Read the model definition and answer for the solid it produces. Units are mm, in the model's axes. A direction names the side the tool comes from. Coordinates: 2 decimals unless noted, no trailing zeros. Order: outer loops, then holes, each group sorted by start corner. A loop starts at its lowest first (then second) coordinate and runs counter-clockwise, first axis right, second up. Notation, with made-up numbers: (11.25, 67) -> (48.25, 67) arc R30 cw to (48.25, 94) -> close; hole circle Ø8 at (66, 75.5). An arc over 180 degrees is marked (long way). Answer in a Markdown table with one row per item.
from build123d import *

# Parameters (mm, degrees)
F0_W     = 25
F0_H     = 6
F1_DEPTH = 100
F2_T     = -2
F3_DEPTH = 2
F4_W     = 27
F4_H     = 10
F5_DEPTH = 2
F6_W     = 60
F6_H     = 32
F7_DEPTH = 2
F6_H_2   = 2
F8_DEPTH = 32


with BuildPart() as f1:
    # F0 (on Right) → F1 (new body)
    with BuildSketch(Plane.YZ):
        Polygon((-49.9118241506, 29.1949231178), (-49.9118241506, -15.4497378229), (30.0881758494, -15.4497378229), (30.0881758494, 64.5502621771), (-14.5564850913, 64.5502621771), align=None)
        with Locations((15.5881758494, -10.4497378229)):
            Rectangle(F0_W, F0_H, mode=Mode.SUBTRACT)
        with Locations((15.5881758494, -10.4497378229)):
            Rectangle(F0_W, F0_H)
    extrude(amount=-F1_DEPTH)

    # F2
    f2_openings = [f1.faces().sort_by_distance(p)[0] for p in [
        (-50, -32.234155, 46.872593),
    ]]
    offset(amount=F2_T, openings=f2_openings)

    # F0 (on Right) → F3 (cut)
    with BuildSketch(Plane.YZ):
        with Locations((15.5881758494, -10.4497378229)):
            Rectangle(F0_W, F0_H)
    extrude(amount=-F3_DEPTH, mode=Mode.SUBTRACT)

    # F4 (on face) → F5 (cut)
    with BuildSketch(Plane(origin=(-100, 0, 0), x_dir=(0, -1, 0), z_dir=(-1, 0, 0))):
        with Locations((-14.5881758494, -8.4497378229)):
            Rectangle(F4_W, F4_H)
    extrude(amount=-F5_DEPTH, mode=Mode.SUBTRACT)

    # F6 (on face) → F7 (cut)
    with BuildSketch(Plane(origin=(0, 30.0881758494, 0), x_dir=(-1, 0, 0), z_dir=(0, 1, 0))):
        with Locations((50, 20.5502621771)):
            Rectangle(F6_W, F6_H)
    extrude(amount=-F7_DEPTH, mode=Mode.SUBTRACT)

    # F6 (on face) → F8 (join)
    with BuildSketch(Plane(origin=(0, 30.0881758494, 0), x_dir=(-1, 0, 0), z_dir=(0, 1, 0))):
        with Locations((50, 3.5502621771)):
            Rectangle(F6_W, F6_H_2)
    extrude(amount=-F8_DEPTH)


solid = f1.part
Q1. Consider line 1 (Z direction, x = -20.5, y = 18); line 2 (X direction, y = 16.5, z = 58); line 3 (Z direction, x = -9, y = -14). Determine where each line is inside the solid, lowest interval first.
Outcome:
| item | result |
|---|---|
| line 1 | -15.45 to -13.45, 2.55 to 4.55, 62.55 to 64.55 |
| line 2 | -100 to -98, -2 to 0 |
| line 3 | -15.45 to -13.45, 62.55 to 64.55 |
Q2. For a pull along X with two mould halves and no side action, classify faces 4 (the face through (-50, 14, 4.55)), 5 (the face through (-49, 30.088, 42)), 6 (the face through (-100, -10, 25)), 7 (the face through (-49, -47.912, 9)) as pulls with the +X half, pulls with the -X half, needs draft (parallel to the pull), parting line crosses it, or undercut.
Outcome:
| item | result |
|---|---|
| face 4 | undercut |
| face 5 | needs draft |
| face 6 | pulls with the -X half |
| face 7 | undercut |
Q3. Given pin 1 (2 mm diameter, centred on y = 8, z = 3.5, fed in from +X); pin 2 (5 mm diameter, centred on x = -27.5, y = -26, fed in from +Z); pin 3 (10 mm diameter, centred on x = -75, z = 50.5, fed in from -Y), each flat-ended and moving along its own axis, determine where each tip first touches the part or whether it passes through.
Outcome:
| item | result |
|---|---|
| pin 1 | x = 0 |
| pin 2 | z = -13.45 |
| pin 3 | y = 28.09 |
Q4. The part is cut by section D-D (z = 11.5). Write down the section's boundary in (x, y), then the cut area to 3 significant figures.
Outcome:
| item | result |
|---|---|
| outline | (-100, -49.91) -> (0, -49.91) -> (0, 30.09) -> (-20, 30.09) -> (-20, 28.09) -> (-2, 28.09) -> (-2, -47.91) -> (-98, -47.91) -> (-98, 28.09) -> (-80, 28.09) -> (-80, 30.09) -> (-100, 30.09) -> close |
| area | 584 mm² |
Q5. For faces 1 (the face through (-49, 6, 62.55)), 2 (the face through (0, -10, 25)), 3 (the face through (-2, -10, 25)), determine the directions among +Z, -Z, +X, -X, +Y, -Y from which every point of the face is accessible in a straight line to the end or side of a thin tool.
Outcome:
| item | result |
|---|---|
| face 1 | -Y |
| face 2 | +Z, -Z, +X, +Y, -Y |
| face 3 | none |
Q6. The part is cut by section C-C (y = 17). Write down the section's boundary in (x, z).
Outcome:
| item | result |
|---|---|
| outline | (-100, -15.45) -> (0, -15.45) -> (0, -13.45) -> (-100, -13.45) -> close; (-100, -3.45) -> (-98, -3.45) -> (-98, 62.55) -> (-2, 62.55) -> (-2, -7.45) -> (0, -7.45) -> (0, 64.55) -> (-100, 64.55) -> close; (-80, 2.55) -> (-20, 2.55) -> (-20, 4.55) -> (-80, 4.55) -> close |
Q7. The part is cut by section A-A (x = -63). Write down the section's boundary in (y, z).
Outcome:
| item | result |
|---|---|
| outline | (-49.91, -15.45) -> (30.09, -15.45) -> (30.09, 4.55) -> (-1.91, 4.55) -> (-1.91, 2.55) -> (28.09, 2.55) -> (28.09, -13.45) -> (-47.91, -13.45) -> (-47.91, 31.19) -> (-49.91, 29.19) -> close; (-16.56, 62.55) -> (28.09, 62.55) -> (28.09, 36.55) -> (30.09, 36.55) -> (30.09, 64.55) -> (-14.56, 64.55) -> close |
Q8. The part is cut by section B-B (y = -10). Write down the section's boundary in (x, z).
Outcome:
| item | result |
|---|---|
| outline | (-100, -15.45) -> (0, -15.45) -> (0, 64.55) -> (-100, 64.55) -> close; hole (-98, -13.45) -> (-2, -13.45) -> (-2, 62.55) -> (-98, 62.55) -> close |
